Here's the drawing with two shaded views (mm, measured from the low corner). I have some questions. A direction names the side the tool comes from. Coordinates: 2 decimals unless noted, no trailing zeros. Order: outer loops, then holes, each group sorted by start corner. A loop starts at its lowest first (then second) coordinate and runs counter-clockwise, first axis right, second up. Notation, with made-up numbers: (31.25, 6) -> (54.25, 6) arc R5 cw to (54.25, 15) -> close; hole circle Ø6 at (60, 68). An arc over 180 degrees is marked (long way). Write item = value, one per line.
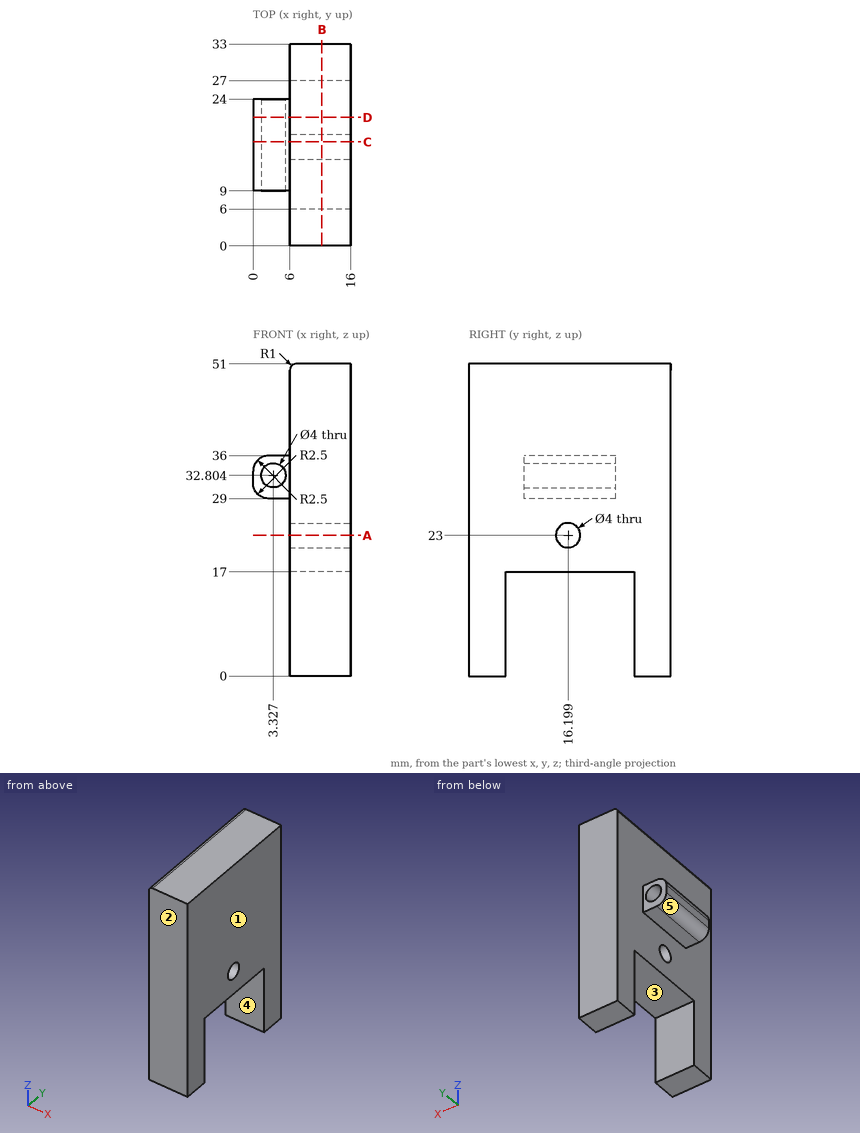
Item 1: For the marked faces 4 and 5, which set-ups out of +Z, -Z, +X, -X, +Y, -Y let a thin tool reach every point of the face, with its end or its side?
A:
face_4 = -Z, +X, -X
face_5 = -Z, -X, +Y, -Y
Item 2: I'm going to push flat-ended pins straight in: P1, Ø4.5, axis at x = 3.33, z = 32.8, coming from the -Y side; P2, Ø1, axis at x = 4, y = 15, coming from the -Z side; P3, Ø4, axis at y = 6, z = 26, coming from the -X side. Where does each tip first touch, or does it pass through?
A:
P1 = 9
P2 = 29
P3 = 6
Item 3: I want a section at B-B, the plane x = 11.25. Please give me the cut outline in (y, z), plus the area to 3 significant figures.
A:
outline = (0, 0) -> (6, 0) -> (6, 17) -> (27, 17) -> (27, 0) -> (33, 0) -> (33, 51) -> (0, 51) -> close; hole circle Ø4 at (16.2, 23)
area = 1,310 mm2
Item 4: If we mould it in two halves opening along Y, with no side actions, what happens to the marked faces 1, 2 and 3? For each: pulls with the +Y half, pulls with the -Y half, needs draft (parallel to the pull), parting line crosses it, or undercut.
A:
face_1 = needs draft
face_2 = pulls with the -Y half
face_3 = undercut
Item 5: I want a section at C-C, the plane y = 17. Please give me the cut outline in (x, z) (1 decimal).
A:
outline = (0, 31.5) arc R2.5 ccw to (2.5, 29) -> (6, 29) -> (6, 24.8) -> (16, 24.8) -> (16, 51) -> (7, 51) arc R1 ccw to (6, 50) -> (6, 36) -> (2.5, 36) arc R2.5 ccw to (0, 33.5) -> close; (6, 17) -> (16, 17) -> (16, 21.2) -> (6, 21.2) -> close; hole circle Ø4 at (3.3, 32.8)
Item 6: I want a section at A-A, the plane z = 23. Please give me the cut outline in (x, y).
A:
outline = (6, 0) -> (16, 0) -> (16, 14.2) -> (6, 14.2) -> close; (6, 18.2) -> (16, 18.2) -> (16, 33) -> (6, 33) -> close
Item 7: If I drill on probe 1 along X at (y, z) = (8, 37.5); probe 2 along Z at (x, y) = (7.25, 23); probe 3 along Z at (x, y) = (2.25, 15.5), over which ranges is the centre line in solid material (lowest first)?
A:
probe_1 = 6 to 16
probe_2 = 17 to 51
probe_3 = 29.01 to 31.12, 34.49 to 35.99
Item 8: I want a section at D-D, the plane y = 21. Please give me the cut outline in (x, z) (1 decimal).
A:
outline = (0, 31.5) arc R2.5 ccw to (2.5, 29) -> (6, 29) -> (6, 17) -> (16, 17) -> (16, 51) -> (7, 51) arc R1 ccw to (6, 50) -> (6, 36) -> (2.5, 36) arc R2.5 ccw to (0, 33.5) -> close; hole circle Ø4 at (3.3, 32.8)
